Autodesk Inventor part; units mm, degrees
ref_plane "YZ Plane" through (0, 0, 0) normal (1, 0, 0) x (0, 1, 0)
ref_plane "XZ Plane" through (0, 0, 0) normal (0, 1, 0) x (-1, 0, 0)
ref_plane "XY Plane" through (0, 0, 0) normal (0, 0, 1) x (1, 0, 0)
sketch "Sketch1" plane through (0, 0, 0) normal (0, 0, 1) x (1, 0, 0)
  circle A0 centre (0, 0) radius 25.4
  dimension "d0" = 50.8
extrude "Can" add sketch "Sketch1" along normal blind 101.6
sketch "Sketch2" plane through (0, 0, 101.6) normal (0, 0, 1) x (1, 0, 0)
  circle A0 centre (0, 0) radius 25.4
  circle A1 centre (-11.049, 0) radius 4.7625
  circle A2 centre (11.049, 0) radius 4.7625
  dimension "d3" = 9.525
  dimension "d4" = 22.098
  dimension "d5" = 11.049
extrude "Studs" add sketch "Sketch2" along normal blind 10.922 contours A1 | A2
thread "Stud 1"
thread "Stud 2"
equation "\"d5\" = 0.5 * d4"
properties part number "Cap"
Could you check a few things on this model? Use its own coordinates, in mm. A direction names the side the tool comes from. Coordinates: 2 decimals unless noted, no trailing zeros. Order: outer loops, then holes, each group sorted by start corner. A loop starts at its lowest first (then second) coordinate and runs counter-clockwise, first axis right, second up. Notation, with made-up numbers: (59.5, 12.5) -> (109.5, 12.5) arc R15 cw to (109.5, 34.5) -> close; hole circle Ø2 at (80.5, 76). An arc over 180 degrees is marked (long way). One line per item, written item: value. Start each with the question number.
1) Imagine slicing it at B-B on x = 0. List the corners of the cut face in (y, z) for me, plus the area to 3 significant figures.
2) Imagine slicing it at A-A on y = 0. List the corners of the cut face in (x, z) for me.
3) Which directions (+Z, -Z, +X, -X, +Y, -Y) give clear straight access to the entire face, cutting with the end or side of a thin tool? Please do faces 1 (the cylindrical face through (-14.828, 2.898, 106.985)), 2 (the flat face through (-11, 0, 112.522)).
4) I'm going to push flat-ended pins straight in: pin 1 (1 mm diameter, centred on y = 19, z = 21, fed in from +X); pin 2 (5 mm diameter, centred on y = 5.5, z = 52.5, fed in from +X); pin 3 (5 mm diameter, centred on x = -19, z = 51, fed in from +Y). Where does each tip first touch, or does it pass through?
5) If I drill on L1, parallel to Z at x = -13, y = 11.5; L2, parallel to X at y = 1, z = 98; L3, parallel to X at y = 7.5, z = 82, over which ranges is the centre line in solid material (lowest first)? Write a range as [from, to].
6) We'd pull the mould along X, two halves only. Please class faces 3 (the cylindrical face through (15.45, 1.82, 106.98)), 4 (the flat face through (11, 0, 112.522)), 5 (the cylindrical face through (-5.506, 24.796, 50.089)): +X half, -X half, draft (parallel to the pull), parting line (faces both ways), or undercut.
7) Imagine slicing it at D-D on x = -8. List the corners of the cut face in (y, z) for me.
8) Imagine slicing it at C-C on z = 74. List the corners of the cut face in (x, y) for me, plus the area to 3 significant figures.
Answer list:
1. outline: (-25.4, 0) -> (25.4, 0) -> (25.4, 101.6) -> (-25.4, 101.6) -> close
1. area: 5,160 mm2
2. outline: (-25.4, 0) -> (25.4, 0) -> (25.4, 101.6) -> (15.81, 101.6) -> (15.81, 112.52) -> (6.29, 112.52) -> (6.29, 101.6) -> (-6.29, 101.6) -> (-6.29, 112.52) -> (-15.81, 112.52) -> (-15.81, 101.6) -> (-25.4, 101.6) -> close
3. face 1: +Z
3. face 2: +Z, +X, -X, +Y, -Y
4. pin 1: stops at x = 17.4
4. pin 2: stops at x = 25.22
4. pin 3: stops at y = 19.31
5. L1: z = [0, 101.6]
5. L2: x = [-25.38, 25.38]
5. L3: x = [-24.27, 24.27]
6. face 3: undercut
6. face 4: draft
6. face 5: parting line
7. outline: (-24.11, 0) -> (24.11, 0) -> (24.11, 101.6) -> (3.66, 101.6) -> (3.66, 112.52) -> (-3.66, 112.52) -> (-3.66, 101.6) -> (-24.11, 101.6) -> close
8. outline: circle Ø50.8 at (0, 0)
8. area: 2,030 mm2
